Input: part model. Units: mm. Frame: model coordinates. Face numbers are marked on the shaded views. A direction names the side the tool comes from. Round coordinates to 2 decimals unless told otherwise and drop trailing zeros. Write each loop counter-clockwise with the first axis right and the second up, starting at its lowest first coordinate (ties: lowest second). Pieces come first, ordered by that corner, then holes. Notation, with made-up numbers: (-27.75, 64) - (9.25, 64) arc R27 cw to (9.25, 92) - close; hole circle Ø5 at (-5, 18). An arc over 180 degrees is marked (long way). Use one line per item in the form item = value.
```python
from build123d import *

# Parameters (mm, degrees)
SKETCH_1_W      = 58.2
SKETCH_1_H      = 58.2
SKETCH_1_W_2    = 53.2
SKETCH_1_H_2    = 53.2
EXTRUDE_1_DEPTH = 22
SKETCH_1_3_W    = 53.2
SKETCH_1_3_H    = 53.2
SKETCH_1_3_R    = 2.55
EXTRUDE_2_DEPTH = 3
FILLET_1_R      = 10


with BuildPart() as part:
    # Sketch 1 → Extrude 1 (new body)
    with BuildSketch(Plane(origin=(0, 0, 0), x_dir=(1, 0, 0), z_dir=(0, 1, 0))):
        Rectangle(SKETCH_1_W, SKETCH_1_H)
        Rectangle(SKETCH_1_W_2, SKETCH_1_H_2, mode=Mode.SUBTRACT)
    extrude(amount=EXTRUDE_1_DEPTH)

    # Sketch 1_3 → Extrude 2 (add)
    with BuildSketch(Plane(origin=(0, 0, 0), x_dir=(1, 0, 0), z_dir=(0, 1, 0))):
        Rectangle(SKETCH_1_3_W, SKETCH_1_3_H)
        with Locations(Location((0, 0, 0), (0, 0, 270))):
            Circle(SKETCH_1_3_R, mode=Mode.SUBTRACT)
    extrude(amount=EXTRUDE_2_DEPTH)

    # Fillet 1
    fillet_1_edges = [part.edges().sort_by_distance(p)[0] for p in [
        (26.6, 12.5, -26.6),
        (-26.6, 12.5, -26.6),
        (-26.6, 12.5, 26.6),
        (26.6, 12.5, 26.6),
        (-29.1, 11, 29.1),
        (29.1, 11, 29.1),
        (29.1, 11, -29.1),
        (-29.1, 11, -29.1),
    ]]
    fillet(fillet_1_edges, radius=FILLET_1_R)


solid = part.part
```
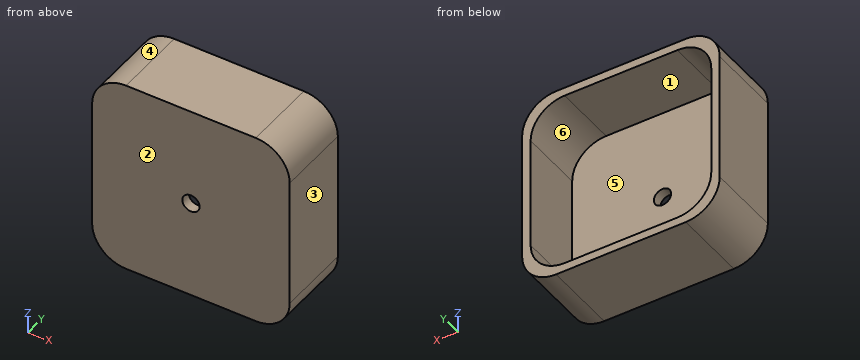
(1) First-contact query: pin 1 Ø4 at (x, z) = (0, 0) entering from +Y; pin 2 Ø16 at (x, z) = (2.5, 11) entering from +Y. Flat tips, straight axial feed; report the tip coordinate or a pass-through.
Derived:
pin_1 = through
pin_2 = 3
(2) Cut plane B-B on z = 0. Output: boundary loops of the cut face in (x, y), then the cut area to 3 significant figures.
Derived:
outline = (-29.1, 0) - (-2.55, 0) - (-2.55, 3) - (-26.6, 3) - (-26.6, 22) - (-29.1, 22) - close; (2.55, 0) - (29.1, 0) - (29.1, 22) - (26.6, 22) - (26.6, 3) - (2.55, 3) - close
area = 254 mm^2
(3) Cut plane D-D on z = -12. Output: boundary loops of the cut face in (x, y), then the cut area to 3 significant figures.
Derived:
outline = (-29.1, 0) - (29.1, 0) - (29.1, 22) - (26.6, 22) - (26.6, 3) - (-26.6, 3) - (-26.6, 22) - (-29.1, 22) - close
area = 270 mm^2
(4) Draft query along X for the marked faces 3, 4, 5 and 6. Return one class per face: released by +X, released by -X, zero draft, split by the parting line, or undercut.
Derived:
face_3 = released by +X
face_4 = released by -X
face_5 = undercut
face_6 = undercut
(5) Access query for the marked faces 1 and 2. Directions: +Z, -Z, +X, -X, +Y, -Y. A direction counts if a zero-diameter tool reaches every point of the face in a straight line with its end or side. Return the directions, or none.
Derived:
face_1 = +Y
face_2 = +Z, -Z, +X, -X, -Y
(6) Cut plane C-C on x = 0. Output: boundary loops of the cut face in (y, z), then the cut area to 3 significant figures.
Derived:
outline = (0, -29.1) - (22, -29.1) - (22, -26.6) - (3, -26.6) - (3, -2.55) - (0, -2.55) - close; (0, 2.55) - (3, 2.55) - (3, 26.6) - (22, 26.6) - (22, 29.1) - (0, 29.1) - close
area = 254 mm^2
(7) Material intervals for L1, parallel to X at y = 14.25, z = -3; L2, parallel to X at y = 1.85, z = 0, sorted ascending.
Derived:
L1 = -29.1 to -26.6, 26.6 to 29.1
L2 = -29.1 to -2.55, 2.55 to 29.1
(8) Cut plane A-A on y = 18.5. Output: boundary loops of the cut face in (x, z), then the cut area to 3 significant figures.
Derived:
outline = (-29.1, -19.1) arc R10 ccw to (-19.1, -29.1) - (19.1, -29.1) arc R10 ccw to (29.1, -19.1) - (29.1, 19.1) arc R10 ccw to (19.1, 29.1) - (-19.1, 29.1) arc R10 ccw to (-29.1, 19.1) - close; hole (-26.6, -16.6) arc R10 ccw to (-16.6, -26.6) - (16.6, -26.6) arc R10 ccw to (26.6, -16.6) - (26.6, 16.6) arc R10 ccw to (16.6, 26.6) - (-16.6, 26.6) arc R10 ccw to (-26.6, 16.6) - close
area = 557 mm^2
